Read the model definition and answer for the solid it produces. Units are mm, in the model's axes. Face numbers are marked on the shaded views. A direction names the side the tool comes from. Coordinates: 2 decimals unless noted, no trailing zeros. Write each loop counter-clockwise with the first axis right and the second up, starting at its lowest first coordinate (ties: lowest second). Pieces come first, ordered by that corner, then holes. Notation, with made-up numbers: (-15.5, -1.75) - (6.5, -1.75) arc R23 ccw to (6.5, 32.25) - close; hole circle Ø11 at (8.25, 73). An arc over 180 degrees is marked (long way). Use a Markdown table: item, result.
from build123d import *

# Parameters (mm, degrees)
BOSS_EXTRUDE1_DEPTH = 18
BOSS_EXTRUDE2_DEPTH = 24.5
CUT_EXTRUDE1_DEPTH  = 17.5
SKETCH6_R           = 12.5
BOSS_EXTRUDE3_DEPTH = 14
BOSS_EXTRUDE4_DEPTH = 3.5
CUT_EXTRUDE6_DEPTH  = 23.5


with BuildPart() as part:
    # Sketch1 → Boss-Extrude1 (new body)
    with BuildSketch(Plane.XY):
        with BuildLine():
            Line((-131.5, -134.5), (131.5, -134.5))
            ThreePointArc((131.5, -134.5), (171.097979746, -118.097979746), (187.5, -78.5))
            Line((187.5, -78.5), (187.5, 78.5))
            ThreePointArc((187.5, 78.5), (171.097979746, 118.097979746), (131.5, 134.5))
            Line((131.5, 134.5), (-131.5, 134.5))
            ThreePointArc((-131.5, 134.5), (-171.097979746, 118.097979746), (-187.5, 78.5))
            Line((-187.5, 78.5), (-187.5, -78.5))
            ThreePointArc((-187.5, -78.5), (-171.097979746, -118.097979746), (-131.5, -134.5))
        make_face()
    extrude(amount=BOSS_EXTRUDE1_DEPTH)

    # Cut-Sweep1: sweep along a path in Sketch3
    with BuildLine(Plane.XY.offset(18)) as cut_sweep1_path:
        Line((131.5, 134.5), (-131.5, 134.5))
        ThreePointArc((-131.5, 134.5), (-171.097979746, 118.097979746), (-187.5, 78.5))
        Line((-187.5, 78.5), (-187.5, -78.5))
        ThreePointArc((-187.5, -78.5), (-171.097979746, -118.097979746), (-131.5, -134.5))
        Line((-131.5, -134.5), (131.5, -134.5))
        ThreePointArc((131.5, -134.5), (171.097979746, -118.097979746), (187.5, -78.5))
        Line((187.5, -78.5), (187.5, 78.5))
        ThreePointArc((187.5, 78.5), (171.097979746, 118.097979746), (131.5, 134.5))
    # Sketch2 → Cut-Sweep1 (sweep, cut)
    with BuildSketch(Plane(origin=(0, 0, 0), x_dir=(0, 0, -1), z_dir=(1, 0, 0))):
        Polygon((-18, 110.392739683), (-10, 134.5), (-18, 134.5), align=None)
    sweep(path=cut_sweep1_path.line, mode=Mode.SUBTRACT)

    # Sketch4 → Boss-Extrude2 (add)
    with BuildSketch(Plane(origin=(0, 0, 0), x_dir=(-1, 0, 0), z_dir=(0, 0, -1))):
        with BuildLine():
            Line((113.5, 96), (-113.5, 96))
            ThreePointArc((-113.5, 96), (-136.127416998, 86.627416998), (-145.5, 64))
            Line((-145.5, 64), (-145.5, -64))
            ThreePointArc((-145.5, -64), (-136.127416998, -86.627416998), (-113.5, -96))
            Line((-113.5, -96), (113.5, -96))
            ThreePointArc((113.5, -96), (136.127416998, -86.627416998), (145.5, -64))
            Line((145.5, -64), (145.5, 64))
            ThreePointArc((145.5, 64), (136.127416998, 86.627416998), (113.5, 96))
        make_face()
    extrude(amount=BOSS_EXTRUDE2_DEPTH)

    # Sketch5 → Cut-Extrude1 (cut)
    with BuildSketch(Plane.XY.offset(18)):
        with BuildLine():
            Line((10.606601718, -78.893398282), (44.72135955, -44.77864045))
            ThreePointArc((44.72135955, -44.77864045), (49.01319592, -32.429470934), (41.987394255, -21.40404767))
            ThreePointArc((41.987394255, -21.40404767), (0, -9.5), (-41.987394255, -21.40404767))
            ThreePointArc((-41.987394255, -21.40404767), (-49.01319592, -32.429470934), (-44.72135955, -44.77864045))
            Line((-44.72135955, -44.77864045), (-10.606601718, -78.893398282))
            ThreePointArc((-10.606601718, -78.893398282), (0, -83.286796564), (10.606601718, -78.893398282))
        make_face()
    extrude(amount=-CUT_EXTRUDE1_DEPTH, mode=Mode.SUBTRACT)

    # Sketch6 → Boss-Extrude3 (add)
    with BuildSketch(Plane.XY.offset(0.5)):
        with Locations((0, -68.286796564)):
            Circle(SKETCH6_R)
    extrude(amount=BOSS_EXTRUDE3_DEPTH)

    # Sketch7 → Boss-Extrude4 (add)
    with BuildSketch(Plane.XY.offset(14.5)):
        with BuildLine():
            Line((-7.459505989, -20.508484033), (-12.129381177, -65.265519969))
            ThreePointArc((-12.129381177, -65.265519969), (0, -80.786796564), (12.129381177, -65.265519969))
            Line((12.129381177, -65.265519969), (7.459505989, -20.508484033))
            ThreePointArc((7.459505989, -20.508484033), (0, -13.786796564), (-7.459505989, -20.508484033))
        make_face()
    extrude(amount=BOSS_EXTRUDE4_DEPTH)

    # Sketch9 → Cut-Extrude6 (cut)
    with BuildSketch(Plane(origin=(0, 0, -24.5), x_dir=(-1, 0, 0), z_dir=(0, 0, -1))):
        with BuildLine():
            Line((113.5, 92.55), (-113.5, 92.55))
            ThreePointArc((-113.5, 92.55), (-133.687898603, 84.187898603), (-142.05, 64))
            Line((-142.05, 64), (-142.05, -64))
            ThreePointArc((-142.05, -64), (-133.687898603, -84.187898603), (-113.5, -92.55))
            Line((-113.5, -92.55), (113.5, -92.55))
            ThreePointArc((113.5, -92.55), (133.687898603, -84.187898603), (142.05, -64))
            Line((142.05, -64), (142.05, 64))
            ThreePointArc((142.05, 64), (133.687898603, 84.187898603), (113.5, 92.55))
        make_face()
    extrude(amount=-CUT_EXTRUDE6_DEPTH, mode=Mode.SUBTRACT)


solid = part.part
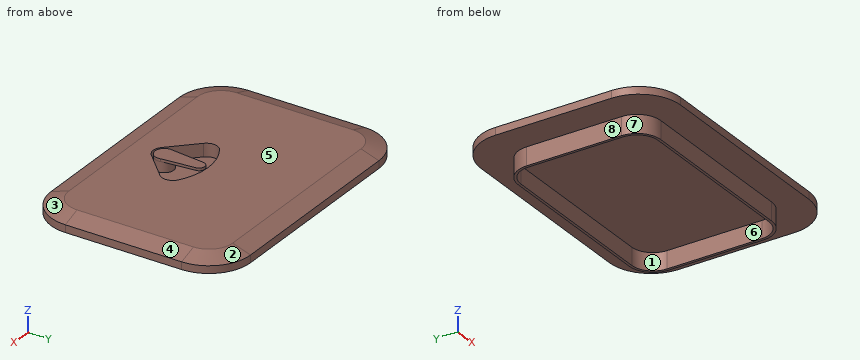
(1) Straight lines are drawn through the part: L1, parallel to X at y = -35, z = -9; L2, parallel to Y at x = 39, z = -14.5; L3, parallel to Z at x = -141.5, y = 102. For each, find the intervals that lie inside material, in ascending order.
Report:
| item | result |
|---|---|
| L1 | x = -145.5 to -142.05, 142.05 to 145.5 |
| L2 | y = -96 to -92.55, 92.55 to 96 |
| L3 | z = 0 to 18 |
(2) Each of these flat-tipped pins is pushed along its axis until it touches: P1, Ø7, axis at x = 26, z = -9, coming from the +Y side; P2, Ø1, axis at x = -125.5, z = -3, coming from the +Y side; P3, Ø7.5, axis at y = 19.5, z = -8, coming from the -X side. Where does it stop, or does it pass through?
Report:
| item | result |
|---|---|
| P1 | stops at y = 96 |
| P2 | stops at y = 93.86 |
| P3 | stops at x = -145.5 |
(3) A cutting plane is placed at C-C, the plane x = -87.5. Write down the section's boundary in (y, z), and give its area (3 significant figures).
Report:
| item | result |
|---|---|
| outline | (-134.5, 0) - (-96, 0) - (-96, -24.5) - (-92.55, -24.5) - (-92.55, -1) - (92.55, -1) - (92.55, -24.5) - (96, -24.5) - (96, 0) - (134.5, 0) - (134.5, 10) - (110.39, 18) - (-110.39, 18) - (-134.5, 10) - close |
| area | 5,000 mm² |
(4) A cutting plane is placed at B-B, the plane x = 0. Write down the section's boundary in (y, z).
Report:
| item | result |
|---|---|
| outline | (-134.5, 0) - (-96, 0) - (-96, -24.5) - (-92.55, -24.5) - (-92.55, -1) - (92.55, -1) - (92.55, -24.5) - (96, -24.5) - (96, 0) - (134.5, 0) - (134.5, 10) - (110.39, 18) - (-9.5, 18) - (-9.5, 0.5) - (-55.79, 0.5) - (-55.79, 14.5) - (-13.79, 14.5) - (-13.79, 18) - (-80.79, 18) - (-80.79, 0.5) - (-83.29, 0.5) - (-83.29, 18) - (-110.39, 18) - (-134.5, 10) - close |
(5) The mould has two halves that part along Y. Classify the marked faces 1, 2, 3 and 4: pulls with the +Y half, pulls with the -Y half, needs draft (parallel to the pull), parting line crosses it, or undercut.
Report:
| item | result |
|---|---|
| face 1 | undercut |
| face 2 | pulls with the +Y half |
| face 3 | pulls with the -Y half |
| face 4 | needs draft |
(6) For the marked faces 5, 6, 7 and 8, determine the directions among +Z, -Z, +X, -X, +Y, -Y from which every point of the face is accessible in a straight line to the end or side of a thin tool.
Report:
| item | result |
|---|---|
| face 5 | +Z, +X, -X, +Y, -Y |
| face 6 | -Z |
| face 7 | -Z, -X, -Y |
| face 8 | -Z, -X, +Y, -Y |
(7) A cutting plane is placed at A-A, the plane y = 15. Write down the section's boundary in (x, z), and give its area (3 significant figures).
Report:
| item | result |
|---|---|
| outline | (-187.5, 0) - (-145.5, 0) - (-145.5, -24.5) - (-142.05, -24.5) - (-142.05, -1) - (142.05, -1) - (142.05, -24.5) - (145.5, -24.5) - (145.5, 0) - (187.5, 0) - (187.5, 10) - (163.39, 18) - (-163.39, 18) - (-187.5, 10) - close |
| area | 7,010 mm² |
